Answer from the drawing. Dimensions are ordinates in mm from the lowest x, y and z of the part. A direction names the side the tool comes from. Round coordinates to 2 decimals unless told otherwise and drop trailing zeros. Order: outer loops, then holes, each group sorted by start corner. A loop starts at its lowest first (then second) coordinate and runs counter-clockwise, first axis right, second up. Notation, with made-up numbers: M -13,38 L 39,38 A29 cw 39,58 Z; hole C 61,88 d6. An arc over 180 degrees is marked long. Answer as a JSON object with one key per item and string values. Group by question number.
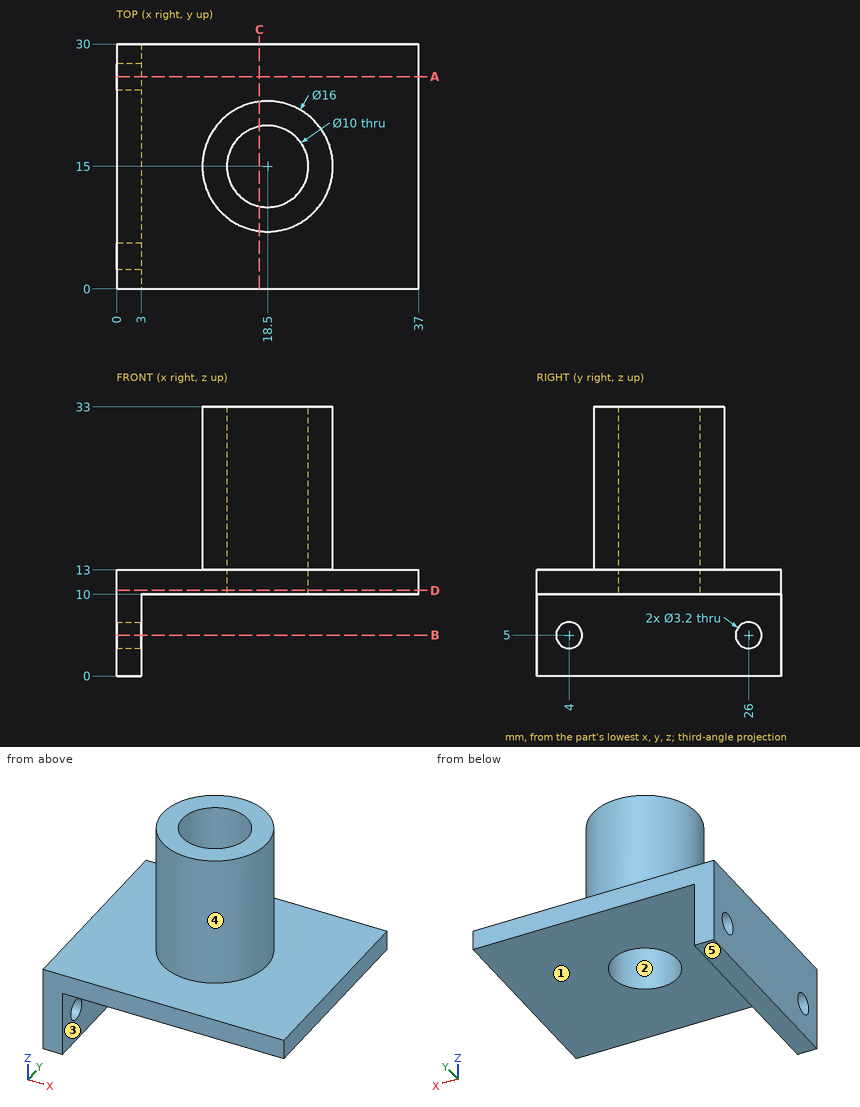
Item 1: The mould has two halves that part along X. Classify the marked faces 1, 2 and 3: +X half, -X half, draft (parallel to the pull), parting line (faces both ways), or undercut.
Item 2: Each of these flat-tipped pins is pushed along its axis until it touches: pin 1 (11.5 mm diameter, centred on x = 18.5, y = 15, fed in from -Z); pin 2 (2 mm diameter, centred on y = 12, z = 22, fed in from +X); pin 3 (4 mm diameter, centred on y = 10.5, z = 29.5, fed in from +X). Where does it stop, or does it pass through?
Item 3: Find section D-D (z = 10.5). Give the vertices of the cut face in (x, y), and give its area (3 significant figures).
Item 4: A tool of negligible diameter and unlimited length cuts with its end or side. For the marked faces 4 and 5, from which of +Z, -Z, +X, -X, +Y, -Y can it reach the whole face along a straight path? Write none if from no direction.
Item 5: Find section C-C (x = 17.5). Give the vertices of the cut face in (y, z).
Item 6: Find section A-A (y = 26). Give the vertices of the cut face in (x, z).
Item 7: Consider L1, parallel to X at y = 5, z = 7; L2, parallel to Z at x = 26.5, y = 11.75; L3, parallel to Y at x = 18.5, z = 28. Determine where each line is inside the solid, lowest interval first.
Item 8: Find section B-B (z = 5). Give the vertices of the cut face in (x, y), and give its area (3 significant figures).
Responses:
{
 "1": {"face 1": "draft", "face 2": "undercut", "face 3": "+X half"},
 "2": {"pin 1": "stops at z = 10", "pin 2": "stops at x = 26.25", "pin 3": "stops at x = 26.1"},
 "3": {"outline": "M 0,0 L 37,0 L 37,30 L 0,30 Z; hole C 18.5,15 d10", "area": "1,030 mm^2"},
 "4": {"face 4": "+Z", "face 5": "-Z, +X, -X, +Y, -Y"},
 "5": {"outline": "M 0,10 L 10.1,10 L 10.1,33 L 7.06,33 L 7.06,13 L 0,13 Z; M 19.9,10 L 30,10 L 30,13 L 22.94,13 L 22.94,33 L 19.9,33 Z"},
 "6": {"outline": "M 0,0 L 3,0 L 3,3.4 L 0,3.4 Z; M 0,6.6 L 3,6.6 L 3,10 L 37,10 L 37,13 L 0,13 Z"},
 "7": {"L1": "x = 0 to 3", "L2": "z = 10 to 13", "L3": "y = 7 to 10, 20 to 23"},
 "8": {"outline": "M 0,0 L 3,0 L 3,2.4 L 0,2.4 Z; M 0,5.6 L 3,5.6 L 3,24.4 L 0,24.4 Z; M 0,27.6 L 3,27.6 L 3,30 L 0,30 Z", "area": "70.8 mm^2"}
}
